```python
from build123d import *

# Parameters (mm, degrees)
F0_R     = 29.21
F1_DEPTH = 69.85
F2_R     = 27.94
F3_DEPTH = 68.834
F4_R     = 1.5875


with BuildPart() as f1:
    # F0 (on Top) → F1 (new body)
    with BuildSketch(Plane.XY):
        Circle(F0_R)
    extrude(amount=F1_DEPTH)

    # F2 (on face) → F3 (cut)
    with BuildSketch(Plane.XY.offset(69.85)):
        Circle(F2_R)
    extrude(amount=-F3_DEPTH, mode=Mode.SUBTRACT)

    # F4
    f4_edges = [f1.edges().sort_by_distance(p)[0] for p in [
        (-27.94, 0, 1.016),
    ]]
    fillet(f4_edges, radius=F4_R)


solid = f1.part
```
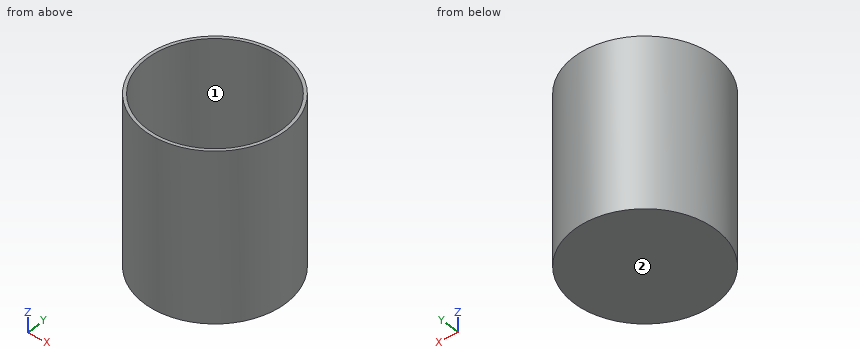
Build history of the part. All positions in model axes, mm. Face numbers are marked on the shaded views. A direction names the side the tool comes from. Coordinates: 2 decimals unless noted, no trailing zeros. Order: outer loops, then holes, each group sorted by start corner. A loop starts at its lowest first (then second) coordinate and runs counter-clockwise, first axis right, second up. Notation, with made-up numbers: (39.5, 88.25) -> (96.5, 88.25) arc R20 cw to (96.5, 122.25) -> close; hole circle Ø9 at (49, 87.5). An arc over 180 degrees is marked (long way). Answer in a Markdown table with one row per item. Add a question column.
Q1. Which spindle directions (+Z, -Z, +X, -X, +Y, -Y) get a long thin tool onto all of the face, cutting with end or side? Do the marked faces 1 and 2. Say none if no direction does.
Q2. Wall check: line 1 along Y through (x, z) = (0, 21.5); line 2 along Z through (x, y) = (-7.5, 23). Give the ranges that are in metal, low to high. Write a range as [from, to].
Q3. Band-saw the part on C-C, the plane z = 54. List the corners of the cut face in (x, y).
Q4. Drop flat-ended pins along their axis: pin 1 (12 mm diameter, centred on x = 12.5, y = 1.5, fed in from +Z); pin 2 (2 mm diameter, centred on x = -17.5, z = 8.5, fed in from -Y); pin 3 (10 mm diameter, centred on x = 0, z = 8, fed in from -Y). Give the stop position or say it passes through.
Answers follow:
| question | item | result |
|---|---|---|
| 1 | face 1 | +Z |
| 1 | face 2 | -Z, +X, -X, +Y, -Y |
| 2 | line 1 | [-29.21, -27.94], [27.94, 29.21] |
| 2 | line 2 | [0, 1.02] |
| 3 | outline | circle Ø58.42 at (0, 0); hole circle Ø55.88 at (0, 0) |
| 4 | pin 1 | z = 1.02 |
| 4 | pin 2 | y = -24.1 |
| 4 | pin 3 | y = -29.21 |
